Geometry check sheet. Reference: the model listing, model coordinates, mm. Face numbers are marked on the shaded views. A direction names the side the tool comes from. Coordinates: 2 decimals unless noted, no trailing zeros. Loops run counter-clockwise (first coordinate to the right, second up) from the corner with the lowest first, then second, coordinate; pieces in that order, holes last. Notation, with made-up numbers: (21.5, -18) - (42.5, -18) arc R25 cw to (42.5, 3) - close; hole circle Ø6 at (31.25, 1). An arc over 180 degrees is marked (long way). One line per item, written item: value.
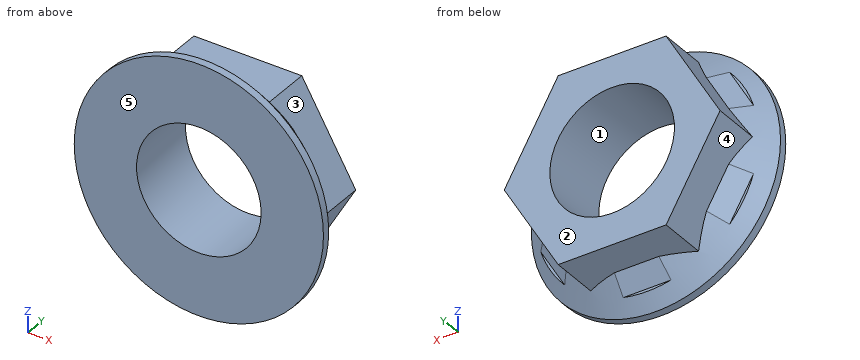
Autodesk Inventor part; units mm, degrees
ref_plane "YZ Plane" through (0, 0, 0) normal (1, 0, 0) x (0, 1, 0)
ref_plane "XZ Plane" through (0, 0, 0) normal (0, 1, 0) x (-1, 0, 0)
ref_plane "XY Plane" through (0, 0, 0) normal (0, 0, 1) x (1, 0, 0)
sketch "Sketch2" plane through (0, 0, 0) normal (0, 1, 0) x (-1, 0, 0)
  circle A0 centre (0, 0) radius 12
  dimension "d3" = 24
extrude "Extrusion1" add sketch "Sketch2" along normal blind 2
sketch "Sketch3" plane through (0, 2, 0) normal (0, 1, 0) x (1, 0, 0)
  line L0 (5.1962, 9) -> (10.3923, 0)
  line L1 (10.3923, 0) -> (5.1962, -9)
  line L2 (5.1962, -9) -> (-5.1962, -9)
  line L3 (-5.1962, -9) -> (-10.3923, 0)
  line L4 (-10.3923, 0) -> (-5.1962, 9)
  line L5 (-5.1962, 9) -> (5.1962, 9)
  point P0 (0, 0)
  point P1 (0, 0)
  dimension "d2" = 18
extrude "Extrusion2" add sketch "Sketch3" along normal blind 5
chamfer "Chamfer1" distance 1.25 angle 45 1 edges at (12, 2, 0)
sketch "Sketch4" plane through (0, 7, 0) normal (0, 1, 0) x (1, 0, 0)
  circle A0 centre (0, 0) radius 6
  dimension "d9" = 12
extrude "Extrusion3" cut sketch "Sketch4" against normal through all
chamfer "Chamfer2" distance 1.5 angle 45 6 edges at (7.7942, 2, 4.5) (7.7942, 2, -4.5) (0, 2, -9) (-7.7942, 2, -4.5) (0, 2, 9) (-7.7942, 2, 4.5)
thread "Thread1"
properties part number "Nylon Nut"
(1) Cross-section at B-B on y = 5. Record the cut outline in (x, z), and give its area (3 significant figures).
Reply:
outline: (-10.39, 0) - (-5.2, -9) - (5.2, -9) - (10.39, 0) - (5.2, 9) - (-5.2, 9) - close; hole circle Ø12 at (0, 0)
area: 167 mm2
(2) Material ranges on probe 1 along Z at (x, y) = (0, 5.5); probe 2 along X at (y, z) = (2.25, 0); probe 3 along X at (y, z) = (6.25, -3.25), recorded low to high. Write a range as from..to.
Reply:
probe 1: -9..-6, 6..9
probe 2: -10.5..-6, 6..10.5
probe 3: -8.52..-5.04, 5.04..8.52
(3) Access from +Z, -Z, +X, -X, +Y, -Y to the whole of each face (thin tool, end or side, straight path). Record for the marked faces 4 and 5.
Reply:
face 4: -Z, -X, +Y
face 5: +Z, -Z, +X, -X, -Y
(4) Go/stop test with flat-tipped pins: pin 1 Ø3 at (x, y) = (5, 2.5) entering from +Z; pin 2 Ø1.4 at (x, y) = (0, 3.5) entering from +Z; pin 3 Ø1.2 at (x, z) = (-9.5, -5) entering from +Y; pin 4 Ø9.5 at (x, z) = (0, 0) entering from -Y. Record where each tip stops, or that it passes through.
Reply:
pin 1: z = 10.76
pin 2: z = 9.7
pin 3: y = 2.37
pin 4: through
(5) Cross-section at A-A on x = 0. Record the cut outline in (y, z), and give its area (3 significant figures).
Reply:
outline: (0, -12) - (0.75, -12) - (2, -10.75) - (2, -10.5) - (3.5, -9) - (7, -9) - (7, -6) - (0, -6) - close; (0, 6) - (7, 6) - (7, 9) - (3.5, 9) - (2, 10.5) - (2, 10.75) - (0.75, 12) - (0, 12) - close
area: 54.7 mm2
(6) Release check for a two-part mould opening along X. For the marked faces 1, 2 and 3 record: pulls with the +X half, pulls with the -X half, needs draft (parallel to the pull), parting line crosses it, or undercut.
Reply:
face 1: undercut
face 2: needs draft
face 3: pulls with the +X half
